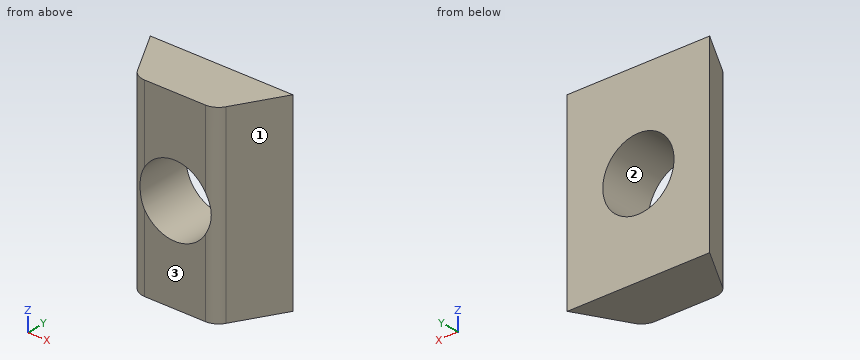
```python
from build123d import *

# Parameters (mm, degrees)
F1_DEPTH    = 12
F3_D        = 4.5
F4_T1_DEPTH = 14.9016126774


# Not quite as in the source:
# - a fillet or chamfer that OpenCascade refuses, or shapes differently, is made with other operations: its cross-section is extruded or revolved along the edge and cut away or added


with BuildPart() as f1:
    # F0 (on Top) → F1 (new body)
    with BuildSketch(Plane.XY):
        Polygon((-2.5, -1.75), (2.5, -1.75), (4.5, 1.75), (-4.5, 1.75), align=None)
    extrude(amount=F1_DEPTH)

    # F3 (through all)
    with Locations(Plane(origin=(0, 1.75, 0), x_dir=(-1, 0, 0), z_dir=(0, 1, 0))):
        with Locations((0, 6)):
            Hole(F3_D / 2)

    # F4: fillet of radius 1 on 2 edges, made by hand

    # F4_s2 → F4_t1 (cut)
    with BuildSketch(Plane.XY.offset(-1.4508063387)):
        with BuildLine():
            ThreePointArc((1.9196774645, -1.75), (2.4216042827, -1.6149100931), (2.7879206067, -1.2461389384))
            Line((2.7879206067, -1.2461389384), (2.5, -1.75))
            Line((2.5, -1.75), (1.9196774645, -1.75))
        make_face()
        with BuildLine():
            ThreePointArc((-1.9196774645, -1.75), (-2.4216042827, -1.6149100931), (-2.7879206067, -1.2461389384))
            Line((-2.7879206067, -1.2461389384), (-2.5, -1.75))
            Line((-2.5, -1.75), (-1.9196774645, -1.75))
        make_face()
    extrude(amount=F4_T1_DEPTH, mode=Mode.SUBTRACT)


solid = f1.part
```
Geometry: final body of the model. Coordinates: model frame, mm. Face numbers are marked on the shaded views. Round coordinates to 2 decimals unless told otherwise and drop trailing zeros. Loops run counter-clockwise (first coordinate to the right, second up) from the corner with the lowest first, then second, coordinate; pieces in that order, holes last. Notation, with made-up numbers: (74.5, 14) -> (91.5, 14) arc R8 ccw to (91.5, 18) -> close; hole circle Ø3 at (16.25, -20). An arc over 180 degrees is marked (long way). Use one line per item in the form item = value. Start each with the question number.
1) First-contact query: P1, Ø1.5, axis at y = 0.5, z = 7, coming from the +X side; P2, Ø2, axis at x = 2, z = 6, coming from the -Y side; P3, Ø4, axis at x = 0, z = 6, coming from the -Y side; P4, Ø1, axis at y = 1, z = 10, coming from the -X side. Flat tips, straight axial feed; report the tip coordinate or a pass-through.
2) Section A-A on x = 0. Output: boundary loops of the cut face in (y, z).
3) Line query: L1, parallel to Z at x = 0, y = -0.6; L2, parallel to Z at x = 2, y = 1; L3, parallel to X at y = -0.15, z = 6. Output: solid intervals per line, ascending.
4) Section D-D on z = 2. Output: boundary loops of the cut face in (x, y), then the cut area to 3 significant figures.
5) Draft query along X for the marked faces 1, 2 and 3. Return one class per face: released by +X, released by -X, zero draft, split by the parting line, or undercut.
6) Section B-B on z = 6.5. Output: boundary loops of the cut face in (x, y), then the cut area to 3 significant figures.
7) Section C-C on y = 0.35. Output: boundary loops of the cut face in (x, z), then the cut area to 3 significant figures.
Response:
q1.P1 = 4.21
q1.P2 = -1.75
q1.P3 = through
q1.P4 = -4.36
q2.outline = (-1.75, 0) -> (1.75, 0) -> (1.75, 3.75) -> (-1.75, 3.75) -> close; (-1.75, 8.25) -> (1.75, 8.25) -> (1.75, 12) -> (-1.75, 12) -> close
q3.L1 = 0 to 3.75, 8.25 to 12
q3.L2 = 0 to 4.97, 7.03 to 12
q3.L3 = -3.41 to -2.25, 2.25 to 3.41
q4.outline = (-4.5, 1.75) -> (-2.79, -1.25) arc R1 ccw to (-1.92, -1.75) -> (1.92, -1.75) arc R1 ccw to (2.79, -1.25) -> (4.5, 1.75) -> close
q4.area = 24.4 mm^2
q5.face_1 = released by +X
q5.face_2 = undercut
q5.face_3 = zero draft
q6.outline = (-4.5, 1.75) -> (-2.79, -1.25) arc R1 ccw to (-2.19, -1.71) -> (-2.19, 1.75) -> close; (2.19, -1.71) arc R1 ccw to (2.79, -1.25) -> (4.5, 1.75) -> (2.19, 1.75) -> close
q6.area = 9.04 mm^2
q7.outline = (-3.7, 0) -> (3.7, 0) -> (3.7, 12) -> (-3.7, 12) -> close; hole circle Ø4.5 at (0, 6)
q7.area = 72.9 mm^2
